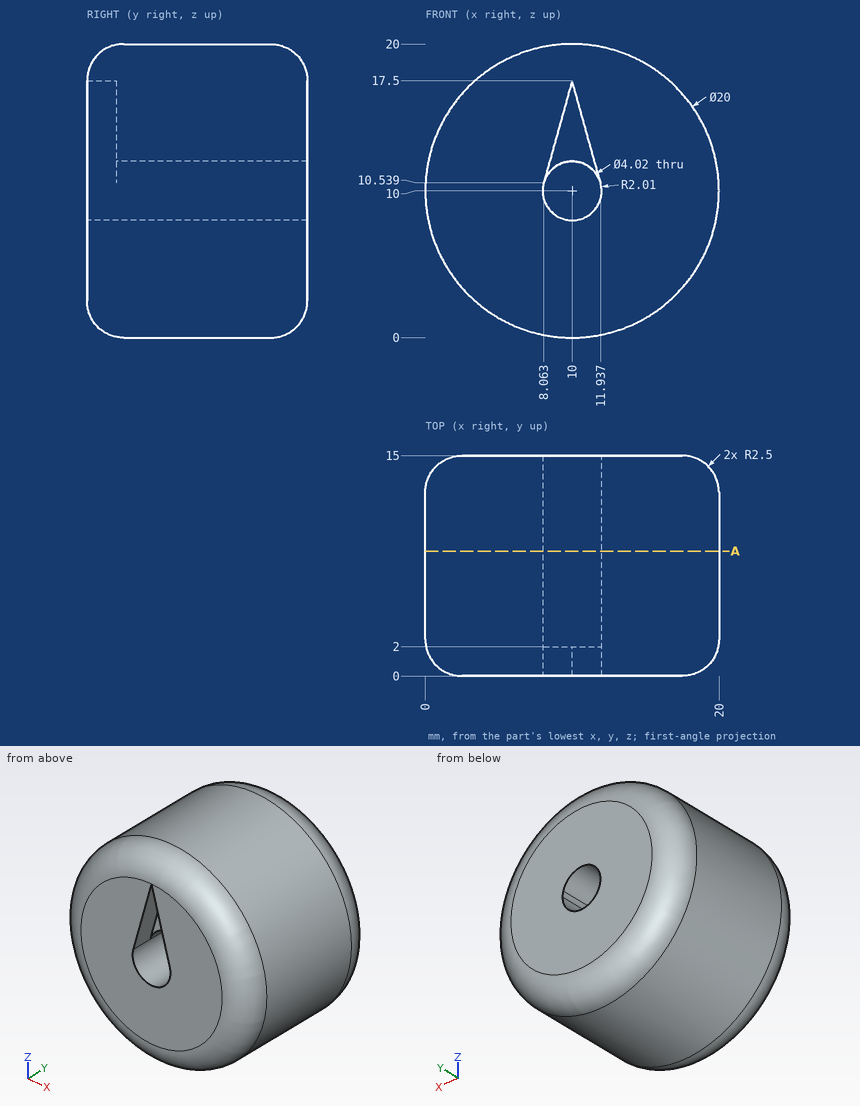
The figure shows three views and two pictorial views of one solid part (mm, origin at its lowest corner). Answer the questions. Round coordinates to 2 decimals unless told otherwise and drop trailing zeros. Write each loop counter-clockwise with the first axis right and the second up, starting at its lowest first coordinate (ties: lowest second). Pieces come first, ordered by that corner, then holes. Notation, with made-up numbers: M -11,80 L 47,80 A19 cw 47,111 Z; hole C 11,10.5 d5. An arc over 180 degrees is marked long. Use a Markdown table: item, result.
1) Flat-ended cylindrical pins translate along their axes: pin 1 (5 mm diameter, centred on x = 5, y = 11.5, fed in from +Z); pin 2 (3 mm diameter, centred on y = 10, z = 3.5, fed in from +X); pin 3 (2 mm diameter, centred on y = 6, z = 9.5, fed in from +X); pin 4 (3 mm diameter, centred on y = 8.5, z = 5.5, fed in from +X). Find the tip coordinate at first contact, or state that the pin passes through.
Answers follow:
| item | result |
|---|---|
| pin 1 | stops at z = 19.68 |
| pin 2 | stops at x = 18.66 |
| pin 3 | stops at x = 20 |
| pin 4 | stops at x = 19.54 |
2) The part is cut by section A-A (y = 8.5). Write down the section's boundary in (x, z).
Answers follow:
| item | result |
|---|---|
| outline | C 10,10 d20; hole M 11.94,10.54 A2.01 ccw long 12.01,10 A2.01 ccw Z |
3) Straight lines are drawn through the part: line 1 along Z through (x, y) = (10, 7); line 2 along Y through (x, z) = (11.25, 2.5); line 3 along Y through (x, z) = (9.75, 16). For each, find the intervals that lie inside material, in ascending order. Write a range as [from, to].
Answers follow:
| item | result |
|---|---|
| line 1 | z = [0, 7.99], [12.01, 20] |
| line 2 | y = [0, 15] |
| line 3 | y = [2, 15] |
